Part model, mm, in its own coordinate system. Face numbers are marked on the shaded views. Round coordinates to 2 decimals unless told otherwise and drop trailing zeros. Loops run counter-clockwise (first coordinate to the right, second up) from the corner with the lowest first, then second, coordinate; pieces in that order, holes last. Notation, with made-up numbers: (80.5, 78.25) -> (95.5, 78.25) arc R28 cw to (95.5, 112.25) -> close; hole circle Ø4 at (8, -37). An arc over 180 degrees is marked (long way). Answer as CSV lines item,"result".
from build123d import *

# Parameters (mm, degrees)
SKETCH1_W               = 66
SKETCH1_H               = 26
BOSS_EXTRUDE1_DEPTH     = 3
BOSS_EXTRUDE2_START     = 3
BOSS_EXTRUDE2_DEPTH     = 3
BOSS_EXTRUDE3_DEPTH     = 10
BOSS_EXTRUDE4_START     = 10
BOSS_EXTRUDE4_DEPTH     = 10
SKETCH2_4_W             = 36
SKETCH2_4_H             = 3
BOSS_EXTRUDE5_DEPTH     = 2.46
SKETCH3_W               = 3
SKETCH3_H               = 2
BOSS_EXTRUDE6_DEPTH     = 2.5
SKETCH4_W               = 11.5
SKETCH4_H               = 10
CUT_EXTRUDE1_DEPTH      = 1
CUT_EXTRUDE1_DEPTH_BACK = 27
M3_CLEARANCE_HOLE1_D    = 3.4
CUT_EXTRUDE2_REACH      = 68
SKETCH8_R               = 5


with BuildPart() as part:
    # Sketch1 → Boss-Extrude1 (new body)
    with BuildSketch(Plane(origin=(0, 0, 0), x_dir=(1, 0, 0), z_dir=(0, 1, 0))):
        Rectangle(SKETCH1_W, SKETCH1_H)
    extrude(amount=BOSS_EXTRUDE1_DEPTH)

    # Sketch1<3> → Boss-Extrude2 (add)
    with BuildSketch(Plane(origin=(0, 0, 0), x_dir=(1, 0, 0), z_dir=(0, 1, 0)).offset(BOSS_EXTRUDE2_START)):
        Polygon((-30, 10), (30, 10), (33, 10), (33, 13), (-33, 13), (-33, -13), (33, -13), (33, -10), (30, -10), (-30, -10), align=None)
    extrude(amount=BOSS_EXTRUDE2_DEPTH)

    # Sketch2 → Boss-Extrude3 (add)
    with BuildSketch(Plane(origin=(0, 6, 0), x_dir=(1, 0, 0), z_dir=(0, 1, 0))):
        Polygon((-3, 10), (-3, 13), (-33, 13), (-33, -13), (-3, -13), (-3, -10), (-30, -10), (-30, 10), align=None)
    extrude(amount=BOSS_EXTRUDE3_DEPTH)

    # Sketch2<3> → Boss-Extrude4 (add)
    with BuildSketch(Plane(origin=(0, 6, 0), x_dir=(1, 0, 0), z_dir=(0, 1, 0)).offset(BOSS_EXTRUDE4_START)):
        Polygon((-30, 10), (-30, 13), (-33, 13), (-33, -13), (-30, -13), (-30, -10), align=None)
    extrude(amount=BOSS_EXTRUDE4_DEPTH)

    # Sketch2<4> → Boss-Extrude5 (add)
    with BuildSketch(Plane(origin=(0, 6, 0), x_dir=(1, 0, 0), z_dir=(0, 1, 0))):
        with Locations((15, 11.5)):
            Rectangle(SKETCH2_4_W, SKETCH2_4_H)
        with Locations((15, -11.5)):
            Rectangle(SKETCH2_4_W, SKETCH2_4_H)
    extrude(amount=BOSS_EXTRUDE5_DEPTH)

    # Sketch3 → Boss-Extrude6 (add)
    with BuildSketch(Plane.XY.offset(-10)):
        with Locations((-0.5, 6.36)):
            Rectangle(SKETCH3_W, SKETCH3_H)
    boss_extrude6 = extrude(amount=BOSS_EXTRUDE6_DEPTH)

    # Mirror1: Boss-Extrude6 across plane
    add(boss_extrude6.mirror(Plane.XY))

    # Sketch4 → Cut-Extrude1 (cut, two sides)
    with BuildSketch(Plane.XZ) as cut_extrude1_sk:
        with Locations((27.25, 0)):
            Rectangle(SKETCH4_W, SKETCH4_H)
    extrude(amount=CUT_EXTRUDE1_DEPTH, mode=Mode.SUBTRACT)
    extrude(cut_extrude1_sk.sketch, amount=-CUT_EXTRUDE1_DEPTH_BACK, mode=Mode.SUBTRACT)

    # M3 Clearance Hole1 (through all)
    with Locations(Plane.XY.offset(13)):
        with Locations((-7.5, 12.5)):
            Hole(M3_CLEARANCE_HOLE1_D / 2)

    # Sketch8 → Cut-Extrude2 (cut, up to next)
    with BuildSketch(Plane.ZY.offset(33), mode=Mode.PRIVATE) as cut_extrude2_sk1:
        with Locations((0, 9)):
            Circle(SKETCH8_R)
    cut_extrude2_tool1 = extrude(cut_extrude2_sk1.sketch, amount=-CUT_EXTRUDE2_REACH, mode=Mode.PRIVATE) & part.part
    add(cut_extrude2_tool1.solids().sort_by_distance((-33, 9, 0))[0], mode=Mode.SUBTRACT)


solid = part.part
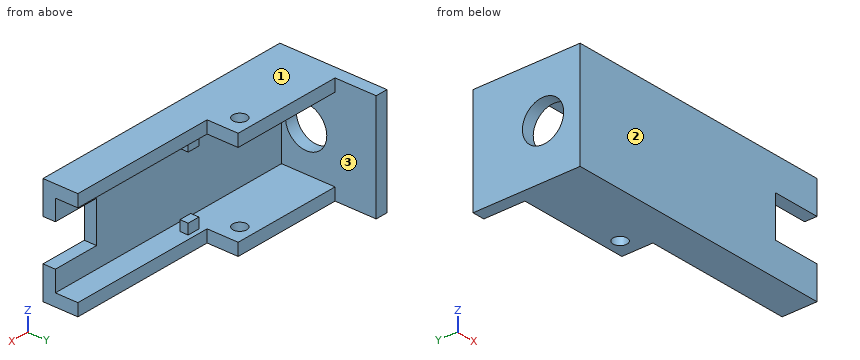
Q1. Drill centre lines: line 1 along Y through (x, z) = (-1, -9.75); line 2 along Y through (x, z) = (-7.5, 11.9); line 3 along Z through (x, y) = (-10, 9). Where is each one in solid material? Low to high.
Geometry results:
line 1,"0 to 3, 5.36 to 7.36"
line 2,"0 to 10.8, 14.2 to 16"
line 3,"-13 to -10, 10 to 13"
Q2. Saw through at D-D, the plane y = 12.5. Write the cut outline in (x, z), then the cut area to 3 significant figures.
Geometry results:
outline,"(-33, -13) -> (-9.2, -13) -> (-9.2, -10) -> (-30, -10) -> (-30, -3.57) -> (-33, -3.57) -> close; (-33, 3.57) -> (-30, 3.57) -> (-30, 10) -> (-9.2, 10) -> (-9.2, 13) -> (-33, 13) -> close; (-5.8, -13) -> (-3, -13) -> (-3, -10) -> (-5.8, -10) -> close; (-5.8, 10) -> (-3, 10) -> (-3, 13) -> (-5.8, 13) -> close"
area,"198 mm2"
Q3. Saw through at C-C, the plane x = -23. Write the cut outline in (y, z), then the cut area to 3 significant figures.
Geometry results:
outline,"(0, -13) -> (16, -13) -> (16, -10) -> (3, -10) -> (3, 10) -> (16, 10) -> (16, 13) -> (0, 13) -> close"
area,"156 mm2"
Q4. Saw through at A-A, the plane z = 0. Write the cut outline in (x, y), then the cut area to 4 significant figures.
Geometry results:
outline,"(-33, 0) -> (21.5, 0) -> (21.5, 3) -> (-30, 3) -> (-30, 4) -> (-33, 4) -> close; (-33, 14) -> (-30, 14) -> (-30, 26) -> (-33, 26) -> close"
area,"202.5 mm2"
Q5. Saw through at B-B, the plane x = -7.5. Write the cut outline in (y, z).
Geometry results:
outline,"(0, -13) -> (10.8, -13) -> (10.8, -10) -> (3, -10) -> (3, 10) -> (10.8, 10) -> (10.8, 13) -> (0, 13) -> close; (14.2, -13) -> (16, -13) -> (16, -10) -> (14.2, -10) -> close; (14.2, 10) -> (16, 10) -> (16, 13) -> (14.2, 13) -> close"
Q6. Drop flat-ended pins along their axis: P1, Ø2, axis at y = 14, z = -5.5, coming from the +X side; P2, Ø1.5, axis at x = -18, z = -11.5, coming from the +Y side; P3, Ø3.5, axis at y = 1, z = 0.5, coming from the +X side. Give the stop position or say it passes through.
Geometry results:
P1,"x = -30"
P2,"y = 16"
P3,"x = 21.5"
Q7. Two-plate mould, pull along Z, no slides. Class the marked faces 1, 2 and 3: pulls with the +Z half, pulls with the -Z half, needs draft (parallel to the pull), parting line crosses it, or undercut.
Geometry results:
face 1,"pulls with the +Z half"
face 2,"needs draft"
face 3,"undercut"
